```python
from build123d import *

# Parameters (mm, degrees)
F0_W     = 73.004455
F0_H     = 61.200289
F1_DEPTH = 34.544
F2_R     = 13.504776
F3_DEPTH = 69.342
F2_R_2   = 21.287393
F4_DEPTH = 25.4


with BuildPart() as f1:
    # F0 (on Front) → F1 (new body)
    with BuildSketch(Plane.XZ):
        with Locations((-15.354115, -8.777854)):
            Rectangle(F0_W, F0_H)
    extrude(amount=-F1_DEPTH)

    # F2 (on face) → F3 (cut)
    with BuildSketch(Plane.XZ):
        with Locations((-16.202834, -9.201426)):
            Circle(F2_R)
    extrude(amount=-F3_DEPTH, mode=Mode.SUBTRACT)

    # F2 (on face) → F4 (join)
    with BuildSketch(Plane.XZ):
        with Locations((-16.202834, -9.201426)):
            Circle(F2_R_2)
        with Locations((-16.202834, -9.201426)):
            Circle(F2_R, mode=Mode.SUBTRACT)
    extrude(amount=F4_DEPTH)


solid = f1.part
```
For this review, take the finished solid that the model builds, in its own axes (mm). A direction names the side the tool comes from. Round coordinates to 2 decimals unless told otherwise and drop trailing zeros. Write each loop counter-clockwise with the first axis right and the second up, starting at its lowest first coordinate (ties: lowest second). Pieces come first, ordered by that corner, then holes. Notation, with made-up numbers: (71, -30.75) - (118, -30.75) arc R3 ccw to (118, -26.75) - close; hole circle Ø6 at (14, -35.75). An arc over 180 degrees is marked (long way). Put each result on its own line as item: value.
Q1. Wall thickness on probe 1 along Z at (x, y) = (-16, 32.5); probe 2 along Y at (x, z) = (16, 8); probe 3 along X at (y, z) = (31.5, -21): over which ranges is each line inside the solid? List them lowest first.
Solved:
probe 1: z = -39.38 to -22.7, 4.3 to 21.82
probe 2: y = 0 to 34.54
probe 3: x = -51.86 to -22.77, -9.63 to 21.15
Q2. We need section C-C (x = 0). Give the boundary of the cut face in (y, z), and give its area (3 significant figures).
Solved:
outline: (-25.4, -23.01) - (0, -23.01) - (0, -39.38) - (34.54, -39.38) - (34.54, 21.82) - (0, 21.82) - (0, 4.61) - (-25.4, 4.61) - close
area: 2,820 mm2
Q3. Insertion check: pin 1 Ø3 at (x, z) = (6, -18.5) entering from -Y; pin 2 Ø12 at (x, z) = (-16.5, -4) entering from +Y; pin 3 Ø1 at (y, z) = (-2, -8) entering from -X; pin 4 Ø10 at (x, y) = (-31.5, -17) entering from +Z. Each pin has a flat end and moves straight along its axis. Give the tip position at first contact, or say it passes through.
Solved:
pin 1: stops at y = 0
pin 2: passes through
pin 3: stops at x = -37.48
pin 4: stops at z = 9.43
Q4. We need section A-A (x = -13). Give the boundary of the cut face in (y, z), and give its area (3 significant figures).
Solved:
outline: (-25.4, -30.25) - (0, -30.25) - (0, -39.38) - (34.54, -39.38) - (34.54, -22.32) - (-25.4, -22.32) - close; (-25.4, 3.92) - (34.54, 3.92) - (34.54, 21.82) - (0, 21.82) - (0, 11.84) - (-25.4, 11.84) - close
area: 1,610 mm2
Q5. We need section B-B (z = -3.5). Give the boundary of the cut face in (x, y), and give its area (3 significant figures).
Solved:
outline: (-51.86, 0) - (-36.71, 0) - (-36.71, -25.4) - (-28.45, -25.4) - (-28.45, 34.54) - (-51.86, 34.54) - close; (-3.96, -25.4) - (4.31, -25.4) - (4.31, 0) - (21.15, 0) - (21.15, 34.54) - (-3.96, 34.54) - close
area: 2,100 mm2
Q6. Machinability: for faces 1 (the face through (-33.1, -12.52, -22.15)), 2 (the face through (-2, -25.4, -9)), which of the approach directions +Z, -Z, +X, -X, +Y, -Y give a long, thin tool a straight path to every point of the face, cutting with its end or side? Answer none if there is none.
Solved:
face 1: -Y
face 2: +Z, -Z, +X, -X, -Y
Q7. We need section D-D (z = 13). Give the boundary of the cut face in (x, y), and give its area (3 significant figures).
Solved:
outline: (-51.86, 0) - (21.15, 0) - (21.15, 34.54) - (-51.86, 34.54) - close
area: 2,520 mm2
